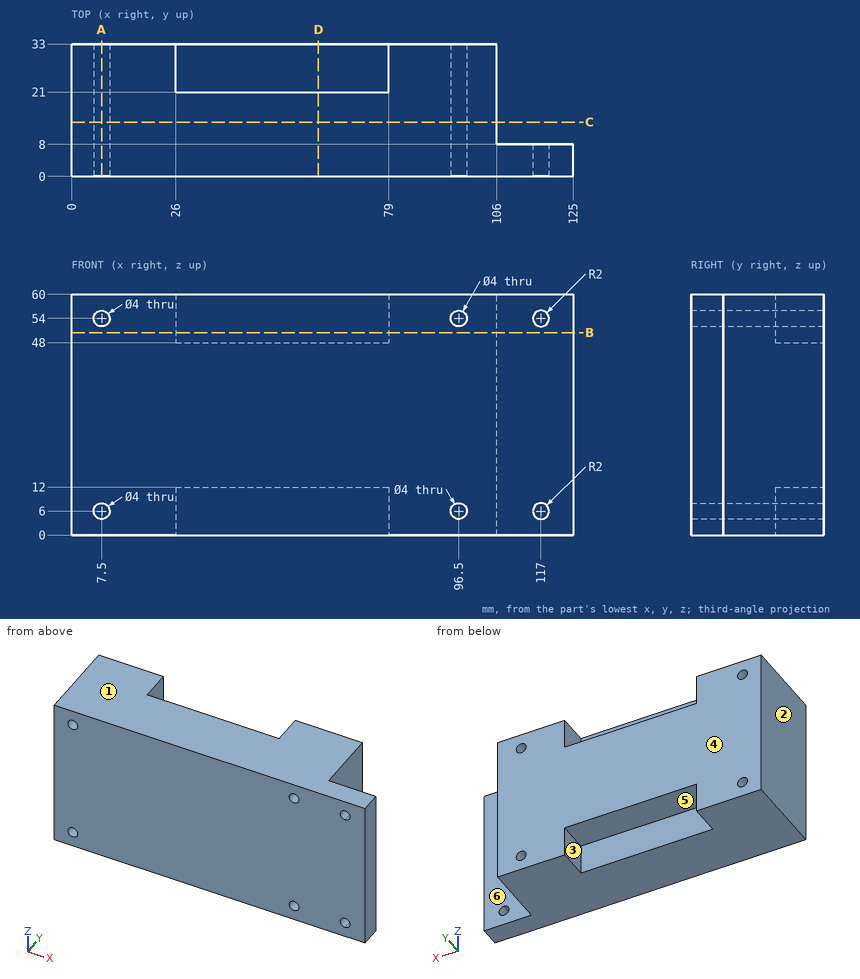
Geometry check sheet. Reference: drawing and pictorial views, mm from the part's lowest x, y, z. A direction names the side the tool comes from. Give positions to 0.01 mm unless a question says otherwise; leave off trailing zeros. Order: outer loops, then holes, each group sorted by start corner. A loop starts at its lowest first (then second) coordinate and runs counter-clockwise, first axis right, second up. Notation, with made-up numbers: M -27.75,7.5 L 22.25,7.5 A23 cw 22.25,23.5 Z; hole C -29.75,-27.75 d6. An arc over 180 degrees is marked long. Return JSON: item names as keys, results as strings. Group by question number.
1) Access from +Z, -Z, +X, -X, +Y, -Y to the whole of each face (thin tool, end or side, straight path). Record for the marked faces 4, 5 and 6.
2) Section check C-C on y = 13.5. Record the cut outline in (x, z).
3) Section check D-D on x = 61.5. Record the cut outline in (y, z), and give its area (3 significant figures).
4) Go/stop test with flat-tipped pins: pin 1 Ø3 at (x, z) = (67, 28.5) entering from -Y; pin 2 Ø6 at (y, z) = (29, 29) entering from +X; pin 3 Ø3.5 at (x, z) = (62, 52.5) entering from +Y; pin 4 Ø5.5 at (x, z) = (118, 30.5) entering from +Y. Record where each tip stops, or that it passes through.
5) Section check A-A on x = 7.5. Record the cut outline in (y, z), and give its area (3 significant figures).
6) Mould release check, pull along X, two halves, no side actions. Record for the marked faces 1, 2 and 3: pulls with the +X half, pulls with the -X half, needs draft (parallel to the pull), parting line crosses it, or undercut.
7) Section check B-B on z = 50.5. Record the cut outline in (x, y), and give its area (3 significant figures).
8) Scan lines: line 1 (Z direction, x = 96.5, y = 14); line 2 (X direction, y = 18, z = 6); line 3 (Z direction, x = 7, y = 10). Record each from-to range of solid material in increasing order.
Answer block:
{
 "1": {"face 4": "+Z, -Z, +X, -X, +Y", "face 5": "-Z, +Y", "face 6": "+Z, -Z, +X, +Y"},
 "2": {"outline": "M 0,0 L 106,0 L 106,60 L 0,60 Z; hole C 7.5,6 d4; hole C 7.5,54 d4; hole C 96.5,6 d4; hole C 96.5,54 d4"},
 "3": {"outline": "M 0,0 L 21,0 L 21,12 L 33,12 L 33,48 L 21,48 L 21,60 L 0,60 Z", "area": "1,690 mm^2"},
 "4": {"pin 1": "stops at y = 0", "pin 2": "stops at x = 106", "pin 3": "stops at y = 21", "pin 4": "stops at y = 8"},
 "5": {"outline": "M 0,0 L 33,0 L 33,4 L 0,4 Z; M 0,8 L 33,8 L 33,52 L 0,52 Z; M 0,56 L 33,56 L 33,60 L 0,60 Z", "area": "1,720 mm^2"},
 "6": {"face 1": "needs draft", "face 2": "pulls with the -X half", "face 3": "undercut"},
 "7": {"outline": "M 0,0 L 125,0 L 125,8 L 106,8 L 106,33 L 79,33 L 79,21 L 26,21 L 26,33 L 0,33 Z", "area": "3,010 mm^2"},
 "8": {"line 1": "z = 0 to 4, 8 to 52, 56 to 60", "line 2": "x = 0 to 5.5, 9.5 to 94.5, 98.5 to 106", "line 3": "z = 0 to 4.06, 7.94 to 52.06, 55.94 to 60"}
}
